Model file for the job. Use its own axes, mm. A direction names the side the tool comes from. Round coordinates to 2 decimals unless told otherwise and drop trailing zeros. Write each loop counter-clockwise with the first axis right and the second up, starting at its lowest first coordinate (ties: lowest second). Pieces come first, ordered by that corner, then holes. Notation, with made-up numbers: (-24.5, -12) - (20.5, -12) arc R5 cw to (20.5, -6) - close; hole circle Ø5 at (57, 65.25). An arc over 180 degrees is marked (long way). Answer as a JSON object with one key per item and string values. Group by question number.
from build123d import *

# Parameters (mm, degrees)
SKETCH3_W                = 13.5
SKETCH3_H                = 5
SKETCH3_W_2              = 10
SKETCH3_W_3              = 5
SKETCH3_H_2              = 23
BOSS_EXTRUDE1_DEPTH      = 45
FILLET1_R                = 2
SKETCH5_R                = 2.1
CUT_EXTRUDE2_DEPTH       = 45
SKETCH6_R                = 2.1
CUT_EXTRUDE3_DEPTH       = 45
SKETCH7_W                = 8.210459319
SKETCH7_H                = 32.58724939
BOSS_EXTRUDE2_DEPTH      = 5
SKETCH8_R                = 2.1
CUT_EXTRUDE5_DEPTH       = 45
BOSS_EXTRUDE3_DEPTH      = 45
SKETCH10_W               = 60.355694637
SKETCH10_H               = 75.381613981
CUT_EXTRUDE7_DEPTH       = 9
SKETCH13_W               = 6.095088126
SKETCH13_H               = 29.055723933
BOSS_EXTRUDE6_DEPTH      = 5
SKETCH14_W               = 6.424633762
SKETCH14_H               = 30.784703445
BOSS_EXTRUDE7_DEPTH      = 5
FILLET3_R                = 2
SKETCH15_R               = 2.1
CUT_EXTRUDE8_DEPTH       = 9
SKETCH16_R               = 2.1
CUT_EXTRUDE9_DEPTH       = 9
SKETCH17_R               = 2.1
SKETCH17_W               = 51.061541061
SKETCH17_H               = 6.00536962
SKETCH17_W_2             = 58.971241115
SKETCH17_H_2             = 35.120826058
CUT_EXTRUDE10_DEPTH      = 42.850344031
CUT_EXTRUDE10_DEPTH_BACK = 29
BOSS_EXTRUDE8_DEPTH      = 5
BOSS_EXTRUDE9_DEPTH      = 5
FILLET5_R                = 4


with BuildPart() as part:
    # Sketch3 → Boss-Extrude1 (new body)
    with BuildSketch(Plane.XY):
        with BuildLine():
            ThreePointArc((-5.06519953, 257.264696919), (-21.146881422, 239.197551787), (-25.551614771, 215.414352888))
            Line((-25.551614771, 215.414352888), (-30.551614771, 215.414352888))
            Line((-30.551614771, 215.414352888), (-30.551614771, 220.414352888))
            ThreePointArc((-30.551614771, 220.414352888), (-24.004098535, 245.112635185), (-5.06519953, 262.264696919))
            Line((-5.06519953, 262.264696919), (-5.06519953, 257.264696919))
        make_face()
        with Locations((1.68480047, 259.764696919)):
            Rectangle(SKETCH3_W, SKETCH3_H)
        with Locations((-35.551614771, 217.914352888)):
            Rectangle(SKETCH3_W_2, SKETCH3_H)
        with Locations((-28.051614771, 203.914352888)):
            Rectangle(SKETCH3_W_3, SKETCH3_H_2)
    extrude(amount=BOSS_EXTRUDE1_DEPTH)

    # Fillet1
    fillet1_edges = [part.edges().sort_by_distance(p)[0] for p in [
        (-40.551614771, 217.914352888, 0),
        (8.43480047, 259.764696919, 45),
        (8.43480047, 259.764696919, 0),
        (-40.551614771, 217.914352888, 45),
    ]]
    fillet(fillet1_edges, radius=FILLET1_R)

    # Sketch5 → Cut-Extrude2 (cut)
    with BuildSketch(Plane(origin=(0, 262.264696919, 0), x_dir=(1, 0, 0), z_dir=(0, 1, 0))):
        with Locations((0.24480047, -40)):
            Circle(SKETCH5_R)
        with Locations((0.24480047, -14.8)):
            Circle(SKETCH5_R)
    extrude(amount=-CUT_EXTRUDE2_DEPTH, mode=Mode.SUBTRACT)

    # Sketch6 → Cut-Extrude3 (cut)
    with BuildSketch(Plane(origin=(0, 220.414352888, 0), x_dir=(1, 0, 0), z_dir=(0, 1, 0))):
        with Locations((-35.551614771, -10)):
            Circle(SKETCH6_R)
        with Locations((-35.551614771, -35)):
            Circle(SKETCH6_R)
    extrude(amount=-CUT_EXTRUDE3_DEPTH, mode=Mode.SUBTRACT)

    # Sketch7 → Boss-Extrude2 (add)
    with BuildSketch(Plane(origin=(0, 262.264696919, 0), x_dir=(1, 0, 0), z_dir=(0, 1, 0))):
        with Locations((1.09445166, -26.923464517)):
            Rectangle(SKETCH7_W, SKETCH7_H)
    extrude(amount=-BOSS_EXTRUDE2_DEPTH)

    # Sketch8 → Cut-Extrude5 (cut)
    with BuildSketch(Plane(origin=(0, 262.264696919, 0), x_dir=(1, 0, 0), z_dir=(0, 1, 0))):
        with Locations((0.24480047, -5)):
            Circle(SKETCH8_R)
        with Locations((0.24480047, -30.2)):
            Circle(SKETCH8_R)
    extrude(amount=-CUT_EXTRUDE5_DEPTH, mode=Mode.SUBTRACT)

    # Sketch9 → Boss-Extrude3 (add, through all)
    with BuildSketch(Plane.XY.offset(45)):
        with BuildLine():
            ThreePointArc((-25.265361734, 225.859750777), (-25.456525287, 224.362535182), (-25.597369426, 222.859750777))
            Line((-25.597369426, 222.859750777), (-18.597369426, 222.859750777))
            Line((-18.597369426, 222.859750777), (-15.597369426, 222.859750777))
            Line((-15.597369426, 222.859750777), (-15.597369426, 247.859750777))
            ThreePointArc((-15.597369426, 247.859750777), (-17.156118075, 245.834377519), (-18.597369426, 243.72377838))
            Line((-18.597369426, 243.72377838), (-18.597369426, 225.859750777))
            Line((-18.597369426, 225.859750777), (-25.265361734, 225.859750777))
        make_face()
        Polygon((-15.597369426, 222.859750777), (-18.597369426, 222.859750777), (-25.551614771, 215.414352888), (-25.551614771, 212.414352888), align=None)
    extrude(amount=-BOSS_EXTRUDE3_DEPTH)

    # Sketch10 → Cut-Extrude7 (cut)
    with BuildSketch(Plane.XY.offset(45)):
        with Locations((-21.743046849, 224.573889929)):
            Rectangle(SKETCH10_W, SKETCH10_H)
    extrude(amount=-CUT_EXTRUDE7_DEPTH, mode=Mode.SUBTRACT)

    # Sketch13 → Boss-Extrude6 (add)
    with BuildSketch(Plane(origin=(0, 220.414352888, 0), x_dir=(1, 0, 0), z_dir=(0, 1, 0))):
        with Locations((-35.175849568, -21.472138034)):
            Rectangle(SKETCH13_W, SKETCH13_H)
    extrude(amount=-BOSS_EXTRUDE6_DEPTH)

    # Sketch14 → Boss-Extrude7 (add)
    with BuildSketch(Plane(origin=(0, 262.264696919, 0), x_dir=(1, 0, 0), z_dir=(0, 1, 0))):
        with Locations((0.1637931, -17.411075239)):
            Rectangle(SKETCH14_W, SKETCH14_H)
    extrude(amount=-BOSS_EXTRUDE7_DEPTH)

    # Fillet3
    fillet3_edges = [part.edges().sort_by_distance(p)[0] for p in [
        (-40.551614771, 217.914352888, 36),
        (8.43480047, 259.764696919, 36),
    ]]
    fillet(fillet3_edges, radius=FILLET3_R)

    # Sketch15 → Cut-Extrude8 (cut)
    with BuildSketch(Plane(origin=(0, 220.414352888, 0), x_dir=(1, 0, 0), z_dir=(0, 1, 0))):
        with Locations((-35.551614771, -8)):
            Circle(SKETCH15_R)
        with Locations((-35.551614771, -28)):
            Circle(SKETCH15_R)
    extrude(amount=-CUT_EXTRUDE8_DEPTH, mode=Mode.SUBTRACT)

    # Sketch16 → Cut-Extrude9 (cut)
    with BuildSketch(Plane(origin=(0, 262.264696919, 0), x_dir=(1, 0, 0), z_dir=(0, 1, 0))):
        with Locations((1.68480047, -8)):
            Circle(SKETCH16_R)
        with Locations((1.68480047, -28)):
            Circle(SKETCH16_R)
    extrude(amount=-CUT_EXTRUDE9_DEPTH, mode=Mode.SUBTRACT)

    # Sketch17 → Cut-Extrude10 (cut, two sides)
    with BuildSketch(Plane(origin=(0, 220.414352888, 0), x_dir=(1, 0, 0), z_dir=(0, 1, 0))) as cut_extrude10_sk:
        with Locations((-35.551614771, -8)):
            Circle(SKETCH17_R)
        with Locations((-15.020844241, 1.00268481)):
            Rectangle(SKETCH17_W, SKETCH17_H)
        with Locations((-11.065994214, -31.560413029)):
            Rectangle(SKETCH17_W_2, SKETCH17_H_2)
    extrude(amount=CUT_EXTRUDE10_DEPTH, mode=Mode.SUBTRACT)
    extrude(cut_extrude10_sk.sketch, amount=-CUT_EXTRUDE10_DEPTH_BACK, mode=Mode.SUBTRACT)

    # Sketch18 → Boss-Extrude8 (add)
    with BuildSketch(Plane.XY.offset(14)):
        with BuildLine():
            ThreePointArc((-15.597369426, 247.859750777), (-10.702470586, 252.977898228), (-5.06519953, 257.264696919))
            Line((-5.06519953, 257.264696919), (8.43480047, 257.264696919))
            Line((8.43480047, 257.264696919), (8.43480047, 262.264696919))
            Line((8.43480047, 262.264696919), (-5.06519953, 262.264696919))
            ThreePointArc((-5.06519953, 262.264696919), (-24.004098535, 245.112635185), (-30.551614771, 220.414352888))
            Line((-30.551614771, 220.414352888), (-40.551614771, 220.414352888))
            Line((-40.551614771, 220.414352888), (-40.551614771, 215.414352888))
            Line((-40.551614771, 215.414352888), (-30.551614771, 215.414352888))
            Line((-30.551614771, 215.414352888), (-30.551614771, 192.414352888))
            Line((-30.551614771, 192.414352888), (-25.551614771, 192.414352888))
            Line((-25.551614771, 192.414352888), (-25.551614771, 212.414352888))
            Line((-25.551614771, 212.414352888), (-15.597369426, 222.859750777))
            Line((-15.597369426, 222.859750777), (-15.597369426, 247.859750777))
        make_face()
        with BuildLine():
            ThreePointArc((-25.551614771, 215.414352888), (-25.728742574, 219.136103908), (-25.597369426, 222.859750777))
            Line((-25.597369426, 222.859750777), (-18.597369426, 222.859750777))
            Line((-18.597369426, 222.859750777), (-25.551614771, 215.414352888))
        make_face(mode=Mode.SUBTRACT)
        with BuildLine():
            ThreePointArc((-25.265361734, 225.859750777), (-22.888422833, 235.14899927), (-18.597369426, 243.72377838))
            Line((-18.597369426, 243.72377838), (-18.597369426, 225.859750777))
            Line((-18.597369426, 225.859750777), (-25.265361734, 225.859750777))
        make_face(mode=Mode.SUBTRACT)
    extrude(amount=BOSS_EXTRUDE8_DEPTH)

    # Sketch19 → Boss-Extrude9 (add)
    with BuildSketch(Plane(origin=(0, 0, 2), x_dir=(-1, 0, 0), z_dir=(0, 0, -1))):
        with BuildLine():
            Line((-8.43480047, 257.264696919), (5.06519953, 257.264696919))
            ThreePointArc((5.06519953, 257.264696919), (10.702470586, 252.977898228), (15.597369426, 247.859750777))
            Line((15.597369426, 247.859750777), (15.597369426, 222.859750777))
            Line((15.597369426, 222.859750777), (25.551614771, 212.414352888))
            Line((25.551614771, 212.414352888), (25.551614771, 192.414352888))
            Line((25.551614771, 192.414352888), (30.551614771, 192.414352888))
            Line((30.551614771, 192.414352888), (30.551614771, 215.414352888))
            Line((30.551614771, 215.414352888), (40.551614771, 215.414352888))
            Line((40.551614771, 215.414352888), (40.551614771, 220.414352888))
            Line((40.551614771, 220.414352888), (30.551614771, 220.414352888))
            ThreePointArc((30.551614771, 220.414352888), (24.004098535, 245.112635185), (5.06519953, 262.264696919))
            Line((5.06519953, 262.264696919), (-8.43480047, 262.264696919))
            Line((-8.43480047, 262.264696919), (-8.43480047, 257.264696919))
        make_face()
        with BuildLine():
            Line((18.597369426, 222.859750777), (25.597369426, 222.859750777))
            ThreePointArc((25.597369426, 222.859750777), (25.728742574, 219.136103908), (25.551614771, 215.414352888))
            Line((25.551614771, 215.414352888), (18.597369426, 222.859750777))
        make_face(mode=Mode.SUBTRACT)
        with BuildLine():
            Line((18.597369426, 225.859750777), (18.597369426, 243.72377838))
            ThreePointArc((18.597369426, 243.72377838), (22.888422833, 235.14899927), (25.265361734, 225.859750777))
            Line((25.265361734, 225.859750777), (18.597369426, 225.859750777))
        make_face(mode=Mode.SUBTRACT)
    extrude(amount=BOSS_EXTRUDE9_DEPTH)

    # Fillet5
    fillet5_edges = [part.edges().sort_by_distance(p)[0] for p in [
        (-40.551614771, 217.914352888, 19),
        (8.43480047, 259.764696919, 19),
        (-40.551614771, 217.914352888, -3),
        (8.43480047, 259.764696919, -3),
    ]]
    fillet(fillet5_edges, radius=FILLET5_R)


solid = part.part
(1) Flat gauge pins, fed straight in: pin 1 (6 mm diameter, centred on y = 201, z = 12.5, fed in from +X); pin 2 (9 mm diameter, centred on y = 237, z = 5, fed in from -X); pin 3 (1 mm diameter, centred on x = -14.5, z = 7, fed in from +Y); pin 4 (8 mm diameter, centred on x = -15, y = 219.5, fed in from -Z). Where does each tip first touch, or does it go through?
(2) 3-axis set-ups, long thin cutter, end or side, ignore diameter. For faces 1 (the flat face through (-33, 215.414, 8)), 2 (the flat face through (-25.552, 203, 8)), 3 (the cylindrical face through (7.23, 259.73, -1.86)): which of +Z, -Z, +X, -X, +Y, -Y reach the whole face in a straight line?
(3) Slice it at C-C (y = 253). Write the cut outline in (x, z).
(4) Slice it at D-D (x = -28). Write the cut outline in (y, z).
(5) Pull direction X, two halves, no side cores. Call faces 4 (the flat face through (-18.597, 235, 8)), 5 (the flat face through (-18, 233, 19)), 6 (the flat face through (-30.552, 204, 8)): pulls with the +X half, pulls with the -X half, needs draft (parallel to the pull), parting line crosses it, or undercut.
(6) Slice it at A-A (z = 8). Write the cut outline in (x, y).
(7) Slice it at B-B (z = 4.75). Write the cut outline in (x, y), then the cut area to 3 significant figures.
(8) Drill centre lines: line 1 (X direction, y = 216.7, z = 8); line 2 (X direction, y = 211.5, z = 11.25); line 3 (X direction, y = 258.4, z = 8). Where is each one in solid material? Low to high. Write a range as from..to.
Answer:
{
 "1": {"pin 1": "x = -25.55", "pin 2": "x = -29.26", "pin 3": "y = 256.59", "pin 4": "z = -3"},
 "2": {"face 1": "+Z, -Z, -X, -Y", "face 2": "+Z, -Z, +X, -Y", "face 3": "-Z, +X, +Y, -Y"},
 "3": {"outline": "(-17.91, -3) - (-10.68, -3) - (-10.68, 19) - (-17.91, 19) - close"},
 "4": {"outline": "(192.41, -3) - (236.7, -3) - (236.7, 19) - (192.41, 19) - close"},
 "5": {"face 4": "undercut", "face 5": "needs draft", "face 6": "pulls with the -X half"},
 "6": {"outline": "(-40.55, 215.41) - (-37.65, 215.41) - (-37.65, 220.41) - (-40.55, 220.41) - close; (-33.45, 215.41) - (-30.55, 215.41) - (-30.55, 192.41) - (-25.55, 192.41) - (-25.55, 212.41) - (-15.6, 222.86) - (-15.6, 247.86) arc R45 cw to (-5.07, 257.26) - (-0.42, 257.26) - (-0.42, 262.26) - (-5.07, 262.26) arc R45 ccw to (-30.55, 220.41) - (-33.45, 220.41) - close; (3.78, 257.26) - (8.43, 257.26) - (8.43, 262.26) - (3.78, 262.26) - close; hole (-25.6, 222.86) arc R45 ccw to (-25.55, 215.41) - (-18.6, 222.86) - close; hole (-25.27, 225.86) - (-18.6, 225.86) - (-18.6, 243.72) arc R45 ccw to start"},
 "7": {"outline": "(-40.55, 215.41) - (-30.55, 215.41) - (-30.55, 192.41) - (-25.55, 192.41) - (-25.55, 212.41) - (-15.6, 222.86) - (-15.6, 247.86) arc R45 cw to (-5.07, 257.26) - (8.43, 257.26) - (8.43, 262.26) - (-5.07, 262.26) arc R45 ccw to (-30.55, 220.41) - (-40.55, 220.41) - close; hole (-25.6, 222.86) arc R45 ccw to (-25.55, 215.41) - (-18.6, 222.86) - close; hole (-25.27, 225.86) - (-18.6, 225.86) - (-18.6, 243.72) arc R45 ccw to start", "area": "616 mm²"},
 "8": {"line 1": "-40.55..-37.65, -33.45..-25.65, -24.35..-21.47", "line 2": "-30.55..-25.55", "line 3": "-11.62..-0.42, 3.78..8.43"}
}
